Geometry check sheet. Reference: the model listing, model coordinates, mm. A direction names the side the tool comes from. Round coordinates to 2 decimals unless told otherwise and drop trailing zeros. Loops run counter-clockwise (first coordinate to the right, second up) from the corner with the lowest first, then second, coordinate; pieces in that order, holes last. Notation, with made-up numbers: M 3.25,24.5 L 16.25,24.5 A25 ccw 16.25,62.5 Z; hole C 80.5,28.5 d1. An arc over 180 degrees is marked long. Answer in a Markdown table with one row per item. Add a question column.
```python
from build123d import *

# Parameters (mm, degrees)
SKETCH1_W           = 68
SKETCH1_H           = 68
BOSS_EXTRUDE1_DEPTH = 7
SKETCH2_W           = 64
SKETCH2_H           = 64
CUT_EXTRUDE1_DEPTH  = 4
SKETCH3_R           = 5.5
CUT_EXTRUDE2_DEPTH  = 2.5


with BuildPart() as part:
    # Sketch1 → Boss-Extrude1 (new body)
    with BuildSketch(Plane(origin=(0, 0, 0), x_dir=(1, 0, 0), z_dir=(0, 1, 0))):
        Rectangle(SKETCH1_W, SKETCH1_H)
    extrude(amount=BOSS_EXTRUDE1_DEPTH)

    # Sketch2 → Cut-Extrude1 (cut)
    with BuildSketch(Plane(origin=(0, 7, 0), x_dir=(1, 0, 0), z_dir=(0, 1, 0))):
        Rectangle(SKETCH2_W, SKETCH2_H)
    extrude(amount=-CUT_EXTRUDE1_DEPTH, mode=Mode.SUBTRACT)

    # Sketch3 → Cut-Extrude2 (cut)
    with BuildSketch(Plane(origin=(0, 3, 0), x_dir=(1, 0, 0), z_dir=(0, 1, 0))):
        with Locations(Location((0, 0, 0), (0, 0, 270))):
            Circle(SKETCH3_R)
    extrude(amount=-CUT_EXTRUDE2_DEPTH, mode=Mode.SUBTRACT)


solid = part.part
```
1) Cross-section at C-C, the plane x = 0. Record the boundary of the cut face in (y, z).
2) Thickness scan on L1, parallel to X at y = 4, z = 30.5; L2, parallel to X at y = 2.3, z = 0. Record the ranges inside material, lowest first. Write a range as [from, to].
3) Cross-section at D-D, the plane z = 0. Record the boundary of the cut face in (x, y).
4) Draft check along X on faces 1 (the flat face through (-32, 5, 0)), 2 (the flat face through (34, 3, 0)), 3 (the flat face through (-34, 3, 0)), 4 (the flat face through (0, 3, -34)). Enter one of: +X half, -X half, draft (parallel to the pull), parting line (faces both ways), or undercut.
5) Go/stop test with flat-tipped pins: pin 1 (17.5 mm diameter, centred on x = 0, z = 0, fed in from +Y); pin 2 (5.5 mm diameter, centred on x = -1.5, z = 1, fed in from +Y). Record where each tip stops, or that it passes through.
6) Cross-section at B-B, the plane x = -19.5. Record the boundary of the cut face in (y, z), plus the area to 3 significant figures.
7) Cross-section at A-A, the plane z = -10.5. Record the boundary of the cut face in (x, y).
8) Set-up check for faces 5 (the flat face through (-3, 7, 33)), 6 (the flat face through (0, 3, -8)): record each of +Z, -Z, +X, -X, +Y, -Y from which the full face is reachable in a straight line by a thin tool's end or side.
Worked answers:
| question | item | result |
|---|---|---|
| 1 | outline | M 0,-34 L 7,-34 L 7,-32 L 3,-32 L 3,-5.5 L 0.5,-5.5 L 0.5,5.5 L 3,5.5 L 3,32 L 7,32 L 7,34 L 0,34 Z |
| 2 | L1 | x = [-34, -32], [32, 34] |
| 2 | L2 | x = [-34, -5.5], [5.5, 34] |
| 3 | outline | M -34,0 L 34,0 L 34,7 L 32,7 L 32,3 L 5.5,3 L 5.5,0.5 L -5.5,0.5 L -5.5,3 L -32,3 L -32,7 L -34,7 Z |
| 4 | face 1 | undercut |
| 4 | face 2 | +X half |
| 4 | face 3 | -X half |
| 4 | face 4 | draft |
| 5 | pin 1 | stops at y = 3 |
| 5 | pin 2 | stops at y = 0.5 |
| 6 | outline | M 0,-34 L 7,-34 L 7,-32 L 3,-32 L 3,32 L 7,32 L 7,34 L 0,34 Z |
| 6 | area | 220 mm2 |
| 7 | outline | M -34,0 L 34,0 L 34,7 L 32,7 L 32,3 L -32,3 L -32,7 L -34,7 Z |
| 8 | face 5 | +Z, -Z, +X, -X, +Y |
| 8 | face 6 | +Y |
